CAD build for the part. Positions are in the model's coordinates, mm. Round coordinates to 2 decimals unless told otherwise and drop trailing zeros.
```python
from build123d import *

# Parameters (mm, degrees)
SKETCH_1_R          = 34
EXTRUDE_1_DEPTH     = 24
SKETCH_2_R          = 7
EXTRUDE_2_DEPTH     = 1.1
SKETCH_3_R          = 6
CUT_EXTRUDE_1_DEPTH = 28.1
SKETCH_4_R          = 1.5
CUT_EXTRUDE_2_DEPTH = 28.1
FILLET_2_R          = 1
FILLET_3_R          = 1


with BuildPart() as part:
    # 草图1 → 凸台-拉伸1 (new body)
    with BuildSketch(Plane.XY):
        Circle(SKETCH_1_R)
    extrude(amount=EXTRUDE_1_DEPTH)

    # 草图2 → 凸台-拉伸2 (add)
    with BuildSketch(Plane(origin=(0, 0, 0), x_dir=(-1, 0, 0), z_dir=(0, 0, -1))):
        Circle(SKETCH_2_R)
    extrude(amount=EXTRUDE_2_DEPTH)

    # 草图3 → 切除-拉伸1 (cut)
    with BuildSketch(Plane(origin=(0, 0, -1.1), x_dir=(-1, 0, 0), z_dir=(0, 0, -1))):
        Circle(SKETCH_3_R)
    extrude(amount=-CUT_EXTRUDE_1_DEPTH, mode=Mode.SUBTRACT)

    # 草图4 → 切除-拉伸2 (cut)
    with BuildSketch(Plane.XY.offset(24)):
        with Locations((0, 22)):
            Circle(SKETCH_4_R)
        with Locations((0, -22)):
            Circle(SKETCH_4_R)
        with Locations((-22, 0)):
            Circle(SKETCH_4_R)
        with Locations((22, 0)):
            Circle(SKETCH_4_R)
        with Locations((0, 15)):
            Circle(SKETCH_4_R)
        with Locations((-15, 0)):
            Circle(SKETCH_4_R)
        with Locations((15, 0)):
            Circle(SKETCH_4_R)
        with Locations((0, -15)):
            Circle(SKETCH_4_R)
    extrude(amount=-CUT_EXTRUDE_2_DEPTH, mode=Mode.SUBTRACT)

    # 圆角2
    fillet_2_edges = [part.edges().sort_by_distance(p)[0] for p in [
        (-34, 0, 0),
    ]]
    fillet(fillet_2_edges, radius=FILLET_2_R)

    # 圆角3
    fillet_3_edges = [part.edges().sort_by_distance(p)[0] for p in [
        (-34, 0, 24),
    ]]
    fillet(fillet_3_edges, radius=FILLET_3_R)


solid = part.part
```
Item 1: Cut at A-A, the plane y = 0. State how many separate pieces and enclosed holes the cut face has, plus the area to 3 significant figures.
Answers follow:
separate pieces: 6
enclosed holes: 0
area: 1,060 mm2
Item 2: Probe line 1 (Y direction, x = 0, z = 18.5); line 2 (Z direction, x = -5.5, y = 27); line 3 (Y direction, x = 15, z = 16). List the from-to ranges inside material, lowest first.
Answers follow:
line 1: y = -34 to -23.5, -20.5 to -16.5, -13.5 to -6, 6 to 13.5, 16.5 to 20.5, 23.5 to 34
line 2: z = 0 to 24
line 3: y = -30.51 to -1.5, 1.5 to 30.51
Item 3: Flat gauge pins, fed straight in: P1, Ø4, axis at x = 15.5, z = 14.5, coming from the -Y side; P2, Ø2.5, axis at x = 0, y = -22, coming from the +Z side; P3, Ø3.5, axis at x = 22, y = 0, coming from the -Z side; P4, Ø6, axis at x = -4.5, z = 13.5, coming from the -Y side. Where does each tip first touch, or does it go through?
Answers follow:
P1: stops at y = -31.2
P2: passes through
P3: stops at z = 0
P4: stops at y = -33.97
Item 4: Two-plate mould, pull along Y, no slides. Class faces 1 (the cylindrical face through (-0.195, -20.513, 12.168)), 2 (the flat face through (-8, 0, 0)), 3 (the cylindrical face through (-6.466, -2.681, -0.542)): released by +Y, released by -Y, zero draft, split by the parting line, or undercut.
Answers follow:
face 1: undercut
face 2: zero draft
face 3: split by the parting line
